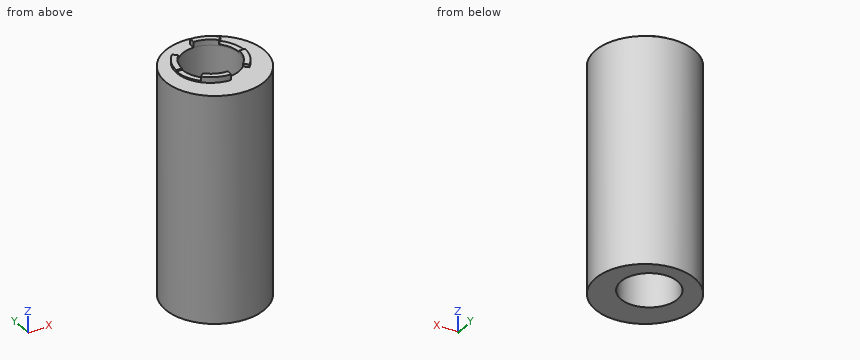
from build123d import *

# Parameters (mm, degrees)
F2_R      = 17.5
F3_DEPTH  = 80
F6_D      = 20
F8_DEPTH  = 2
F10_DEPTH = 0.5
F12_DEPTH = 1


with BuildPart() as f3:
    # F2 (on Top) → F3 (new body)
    with BuildSketch(Plane.XY):
        Circle(F2_R)
    extrude(amount=F3_DEPTH)

    # F6 (through all)
    with Locations(Plane.XY.offset(80)):
        with Locations((0, 2.5)):
            Hole(F6_D / 2)

    # F7 (on offset) → F8 (join)
    with BuildSketch(Plane.XY.offset(80)):
        with BuildLine():
            Line((0, -9.5), (0, -7.5))
            ThreePointArc((0, -7.5), (-3.8268343237, -6.7387953251), (-7.0710678119, -4.5710678119))
            Line((-7.0710678119, -4.5710678119), (-8.4852813742, -5.9852813742))
            ThreePointArc((-8.4852813742, -5.9852813742), (-4.5922011884, -8.5865543901), (0, -9.5))
        make_face()
        with BuildLine():
            Line((0, 14.4321346406), (0, 12.5))
            ThreePointArc((0, 12.5), (3.8268343237, 11.7387953251), (7.0710678119, 9.5710678119))
            Line((7.0710678119, 9.5710678119), (8.4852813742, 10.9852813742))
            ThreePointArc((8.4852813742, 10.9852813742), (4.5922011884, 13.5865543901), (0, 14.5))
            Line((0, 14.5), (0, 14.4321346406))
        make_face()
    extrude(amount=F8_DEPTH)

    # F9 (on offset) → F10 (join)
    with BuildSketch(Plane.XY.offset(80)):
        with BuildLine():
            Line((-8.4852813742, -5.9852813742), (-7.0710678119, -4.5710678119))
            ThreePointArc((-7.0710678119, -4.5710678119), (-9.2387953251, -1.3268343237), (-10, 2.5))
            Line((-10, 2.5), (-12, 2.5))
            ThreePointArc((-12, 2.5), (-11.0865543901, -2.0922011884), (-8.4852813742, -5.9852813742))
        make_face()
        with BuildLine():
            Line((8.4328658848, 10.9328658848), (7.0710678119, 9.5710678119))
            ThreePointArc((7.0710678119, 9.5710678119), (9.2387953251, 6.3268343237), (10, 2.5))
            Line((10, 2.5), (12, 2.5))
            ThreePointArc((12, 2.5), (11.0865543901, 7.0922011884), (8.4852813742, 10.9852813742))
            Line((8.4852813742, 10.9852813742), (8.4328658848, 10.9328658848))
        make_face()
    extrude(amount=F10_DEPTH)

    # F11 (on offset) → F12 (join)
    with BuildSketch(Plane.XY.offset(80)):
        with BuildLine():
            Line((-12, 2.5), (-10, 2.5))
            ThreePointArc((-10, 2.5), (-9.2387953251, 6.3268343237), (-7.0710678119, 9.5710678119))
            Line((-7.0710678119, 9.5710678119), (-8.4852813742, 10.9852813742))
            ThreePointArc((-8.4852813742, 10.9852813742), (-11.0865543901, 7.0922011884), (-12, 2.5))
        make_face()
        with BuildLine():
            Line((12, 2.5), (10, 2.5))
            ThreePointArc((10, 2.5), (9.2387953251, -1.3268343237), (7.0710678119, -4.5710678119))
            Line((7.0710678119, -4.5710678119), (8.4852813742, -5.9852813742))
            ThreePointArc((8.4852813742, -5.9852813742), (11.0865543901, -2.0922011884), (12, 2.5))
        make_face()
    extrude(amount=F12_DEPTH)


solid = f3.part
Source: CAD feature listing. Evaluate the final solid. Frame: model axes, mm. Round coordinates to 2 decimals unless told otherwise and drop trailing zeros. Loops run counter-clockwise (first coordinate to the right, second up) from the corner with the lowest first, then second, coordinate; pieces in that order, holes last. Notation, with made-up numbers: (-37.75, 15) -> (-20.75, 15) arc R33 ccw to (-20.75, 43) -> close; hole circle Ø4 at (-26.75, 10). An arc over 180 degrees is marked (long way). Answer as a JSON object with one key per item and string values. Group by question number.
Q1. Section query A-A (y = 5). Output: boundary loops of the cut face in (x, z), plus the area to 3 significant figures.
Q2. Ray query, line 1 (Y direction, x = 0, z = 39); line 2 (Z direction, x = 13, y = 9); line 3 (Y direction, x = 8.5, z = 65.5). Return the intervals inside material, ascending. Write a range as from..to.
Q3. Section query D-D (y = 0). Output: boundary loops of the cut face in (x, z), plus the area to 3 significant figures.
Q4. Section query B-B (x = -3). Output: boundary loops of the cut face in (y, z), plus the area to 3 significant figures.
Q5. Section query C-C (z = 41). Output: boundary loops of the cut face in (x, y).
Q6. Contact query for flat-ended pins moving along their axis: P1, Ø8, axis at x = 1.5, y = 10, coming from the -Z side; P2, Ø1.5, axis at x = 9, y = -2.5, coming from the +Z side; P3, Ø2.5, axis at x = -10, y = 0, coming from the +Z side; P4, Ø1.5, axis at x = 8.5, y = 6, coming from the +Z side. Output: stop coordinate, or through.
Completed:
{
 "1": {"outline": "(-16.77, 0) -> (-9.68, 0) -> (-9.68, 81) -> (-11.74, 81) -> (-11.74, 80) -> (-16.77, 80) -> close; (9.68, 0) -> (16.77, 0) -> (16.77, 80) -> (11.74, 80) -> (11.74, 80.5) -> (9.68, 80.5) -> close", "area": "1,140 mm²"},
 "2": {"line 1": "-17.5..-7.5, 12.5..17.5", "line 2": "0..80", "line 3": "-15.3..-2.77, 7.77..15.3"},
 "3": {"outline": "(-17.5, 0) -> (-9.68, 0) -> (-9.68, 80.5) -> (-11.74, 80.5) -> (-11.74, 80) -> (-17.5, 80) -> close; (9.68, 0) -> (17.5, 0) -> (17.5, 80) -> (11.74, 80) -> (11.74, 81) -> (9.68, 81) -> close", "area": "1,250 mm²"},
 "4": {"outline": "(-17.24, 0) -> (-7.04, 0) -> (-7.04, 82) -> (-9.12, 82) -> (-9.12, 80) -> (-17.24, 80) -> close; (12.04, 0) -> (17.24, 0) -> (17.24, 80) -> (12.04, 80) -> close", "area": "1,240 mm²"},
 "5": {"outline": "circle Ø35 at (0, 0); hole circle Ø20 at (0, 2.5)"},
 "6": {"P1": "z = 0", "P2": "z = 81", "P3": "z = 80.5", "P4": "through"}
}
